from build123d import *

# Parameters (mm, degrees)
F0_W      = 220
F0_H      = 160
F1_DEPTH  = 2
F3_DEPTH  = 25
F4_W      = 24
F4_H      = 5
F5_DEPTH  = 60
F6_R      = 5
F7_DEPTH  = 25
F8_W      = 24
F8_H      = 5
F9_DEPTH  = 60
F10_R     = 4
F11_DEPTH = 25
F12_DEPTH = 100


with BuildPart() as f1:
    # F0 (on Top) → F1 (new body)
    with BuildSketch(Plane.XY):
        with Locations((-70.886021, -4.76821)):
            Rectangle(F0_W, F0_H)
    extrude(amount=-F1_DEPTH)

    # F2 (on face) → F3 (cut)
    with BuildSketch(Plane.XY):
        with BuildLine():
            Line((12.277737, -5), (12.277737, 5))
            Line((12.277737, 5), (-147.722263, 5))
            ThreePointArc((-147.722263, 5), (-152.722263, 0), (-147.722263, -5))
            Line((-147.722263, -5), (12.277737, -5))
        make_face()
    extrude(amount=-F3_DEPTH, mode=Mode.SUBTRACT)

    # F4 (on face) → F5 (join)
    with BuildSketch(Plane.XY):
        with Locations((-67.722263, -9.5)):
            Rectangle(F4_W, F4_H)
        with Locations((-67.722263, 9.5)):
            Rectangle(F4_W, F4_H)
    extrude(amount=F5_DEPTH)

    # F6 (on face) → F7 (cut)
    with BuildSketch(Plane.XZ.offset(12)):
        with Locations((-67.722263, 49)):
            Circle(F6_R)
    extrude(amount=-F7_DEPTH, mode=Mode.SUBTRACT)

    # F8 (on face) → F9 (join)
    with BuildSketch(Plane.XY):
        with Locations((-19.722263, -19)):
            Rectangle(F8_W, F8_H)
        with Locations((-19.722263, -67.5)):
            Rectangle(F8_W, F8_H)
    extrude(amount=F9_DEPTH)

    # F10 (on face) → F11 (cut)
    with BuildSketch(Plane.XZ.offset(21.5)):
        with Locations((-19.722263, 49)):
            Circle(F10_R)
    extrude(amount=-F11_DEPTH, mode=Mode.SUBTRACT)

    # F10 (on face) → F12 (cut)
    with BuildSketch(Plane.XZ.offset(21.5)):
        with Locations((-19.722263, 49)):
            Circle(F10_R)
    extrude(amount=F12_DEPTH, mode=Mode.SUBTRACT)


solid = f1.part
Could you check a few things on this model? Use its own coordinates, in mm. A direction names the side the tool comes from. Coordinates: 2 decimals unless noted, no trailing zeros. Order: outer loops, then holes, each group sorted by start corner. A loop starts at its lowest first (then second) coordinate and runs counter-clockwise, first axis right, second up.
Q1. Suppose I cut it at D-D on z = 49. Give the number of separate pieces and of enclosed holes in the cut face, and give its area (3 significant figures).
Q2. Which directions (+Z, -Z, +X, -X, +Y, -Y) give clear straight access to the entire face, cutting with the end or side of a thin tool? Please do faces 1 (the flat face through (-68, -12, 30)), 2 (the cylindrical face through (-152.72, 0.11, -0.99)), 3 (the flat face through (-7.722, -68, 30)), 4 (the flat face through (-31.722, -19, 30)), 5 (the flat face through (-20, -65, 30)).
Q3. Thinking about a two-plate mould opening in Y: for faces 6 (the flat face through (-20, -21.5, 30)), 7 (the flat face through (-55.722, 9, 30)), 8 (the flat face through (-68, 12, 30)), which applies, released by +Y, released by -Y, zero draft, split by the parting line, or undercut?
Q4. Suppose I cut it at B-B on z = 33. Please give me the cut outline in (x, y).
Q5. Please list where these lines run through material, in increasing order: L1, parallel to X at y = -68.45, z = 49; L2, parallel to Z at x = -53, y = 20.5; L3, parallel to Y at x = -25, z = 17.5.
Q6. Suppose I cut it at C-C on x = -144. Please give me the cut outline in (y, z), and give its area (3 significant figures).
Q7. Will these pins go through, and if not, where does the flat tip stop? pin 1 (7 mm diameter, centred on x = -63.5, z = 27.5, fed in from +Y); pin 2 (12 mm diameter, centred on x = -23, z = 24.5, fed in from +Y); pin 3 (6 mm diameter, centred on x = 14.5, y = -13.5, fed in from +Z); pin 4 (8 mm diameter, centred on x = -67.72, z = 49, fed in from +Y).
Q8. Suppose I cut it at A-A on y = 0. Please give me the cut outline in (x, z).
Answer:
1. separate pieces: 8
1. enclosed holes: 0
1. area: 300 mm2
2. face 1: +Z, +X, -X, -Y
2. face 2: +Z, -Z
2. face 3: +Z, +X, +Y, -Y
2. face 4: +Z, -X, +Y, -Y
2. face 5: +Z, +X, -X
3. face 6: undercut
3. face 7: zero draft
3. face 8: released by +Y
4. outline: (-79.72, -12) - (-55.72, -12) - (-55.72, -7) - (-79.72, -7) - close; (-79.72, 7) - (-55.72, 7) - (-55.72, 12) - (-79.72, 12) - close; (-31.72, -70) - (-7.72, -70) - (-7.72, -65) - (-31.72, -65) - close; (-31.72, -21.5) - (-7.72, -21.5) - (-7.72, -16.5) - (-31.72, -16.5) - close
5. L1: x = -31.72 to -23.72, -15.72 to -7.72
5. L2: z = -2 to 0
5. L3: y = -70 to -65, -21.5 to -16.5
6. outline: (-84.77, -2) - (-5, -2) - (-5, 0) - (-84.77, 0) - close; (5, -2) - (75.23, -2) - (75.23, 0) - (5, 0) - close
6. area: 300 mm2
7. pin 1: stops at y = 12
7. pin 2: stops at y = -16.5
7. pin 3: stops at z = 0
7. pin 4: passes through
8. outline: (-180.89, -2) - (-152.72, -2) - (-152.72, 0) - (-180.89, 0) - close; (12.28, -2) - (39.11, -2) - (39.11, 0) - (12.28, 0) - close
